Geometry check sheet. Reference: the model listing, model coordinates, mm. Give positions to 0.01 mm unless a question says otherwise; leave off trailing zeros. Loops run counter-clockwise (first coordinate to the right, second up) from the corner with the lowest first, then second, coordinate; pieces in that order, holes last. Notation, with made-up numbers: (85.25, -8.75) -> (105.25, -8.75) arc R22 cw to (105.25, 29.25) -> close; hole circle Ø1 at (3.25, 76). An arc over 180 degrees is marked (long way). Write each question's results on one line, items separated by ' | '. Start each with the question number.
1) Sectioned sample at C-C on y = -150.5. Record the cut outline in (x, z), then the cut area to 3 significant figures.
2) Sectioned sample at B-B on x = 0. Record the cut outline in (y, z), then the cut area to 3 significant figures.
3) Sectioned sample at D-D on x = -48.5. Record the cut outline in (y, z).
4) Depth check by flat-ended pin: pin 1 (4 mm diameter, centred on x = 31.5, z = 4.5, fed in from +Y); pin 2 (8 mm diameter, centred on x = 16, z = -1, fed in from -Y); pin 3 (8 mm diameter, centred on x = 31, z = -3, fed in from +Y). Enter the tip coordinate at first touch or a pass-through.
5) Scan lines: line 1 (Y direction, x = 6.5, z = -0.5); line 2 (X direction, y = 9.5, z = 6.5); line 3 (X direction, y = 141, z = -0.75). Record each from-to range of solid material in increasing order. Write a range as from..to.
6) Sectioned sample at A-A on z = 0. Record the cut outline in (x, y).
```python
from build123d import *

# Parameters (mm, degrees)
F0_R     = 8
F0_R_2   = 6
F1_DEPTH = 185
F2_R     = 6
F4_DEPTH = 50
F3_R     = 6
F5_DEPTH = 25
F6_R     = 3.75
F7_DEPTH = 100


with BuildPart() as f1:
    # F0 (on Front) → F1 (new body, symmetric)
    with BuildSketch(Plane.XZ):
        Circle(F0_R)
        Circle(F0_R_2, mode=Mode.SUBTRACT)
        Circle(F0_R_2)
    extrude(amount=F1_DEPTH, both=True)

    # F2 (on face) → F4 (join)
    with BuildSketch(Plane.XZ.offset(185)):
        Circle(F2_R)
    extrude(amount=F4_DEPTH)

    # F3 (on face) → F5 (join)
    with BuildSketch(Plane(origin=(0, 185, 0), x_dir=(-1, 0, 0), z_dir=(0, 1, 0))):
        Circle(F3_R)
    extrude(amount=F5_DEPTH)

    # F6 (on Right) → F7 (join, symmetric)
    with BuildSketch(Plane.YZ):
        with Locations((-227.5, 0)):
            Circle(F6_R)
    extrude(amount=F7_DEPTH, both=True)


solid = f1.part
```
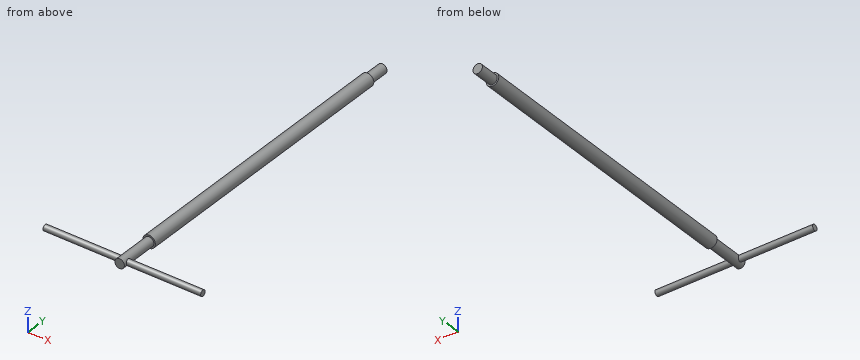
Result:
1) outline: circle Ø16 at (0, 0) | area: 201 mm^2
2) outline: (-235, -6) -> (-185, -6) -> (-185, -8) -> (185, -8) -> (185, -6) -> (210, -6) -> (210, 6) -> (185, 6) -> (185, 8) -> (-185, 8) -> (-185, 6) -> (-235, 6) -> close | area: 6,820 mm^2
3) outline: circle Ø7.5 at (-227.5, 0)
4) pin 1: y = -224.7 | pin 2: y = -231.25 | pin 3: y = -223.75
5) line 1: -231.22..-223.78, -185..185 | line 2: -4.66..4.66 | line 3: -7.96..7.96
6) outline: (-100, -231.25) -> (-6, -231.25) -> (-6, -235) -> (6, -235) -> (6, -231.25) -> (100, -231.25) -> (100, -223.75) -> (6, -223.75) -> (6, -185) -> (8, -185) -> (8, 185) -> (6, 185) -> (6, 210) -> (-6, 210) -> (-6, 185) -> (-8, 185) -> (-8, -185) -> (-6, -185) -> (-6, -223.75) -> (-100, -223.75) -> close
